Here's how the part is built. I have some questions about the finished solid (model axes, mm). Face numbers are marked on the shaded views. A direction names the side the tool comes from. Give positions to 0.01 mm unless a question says otherwise; leave off trailing zeros. Loops run counter-clockwise (first coordinate to the right, second up) from the corner with the lowest first, then second, coordinate; pieces in that order, holes last.
Q1. If we section it at B-B (z = 44.5): Please give me the cut outline in (x, y).
Q2. If we section it at C-C (x = 3): Please give me the cut outline in (y, z), plus the area to 3 significant figures.
Q3. I need wall thicknesses on line 1 (Z direction, x = 9.25, y = -12); line 2 (Y direction, x = 1.25, z = 5.5); line 3 (Y direction, x = 0.5, z = 43). Which ranges of each line are inside material? Lowest first, please.
Q4. Will these pins go through, and if not, where does the flat tip stop? P1, Ø3.5, axis at x = 7.5, z = -3, coming from the -Y side; P2, Ø5, axis at x = 8.5, z = 4.5, coming from the +Y side; P3, Ø3.5, axis at x = 0.5, z = -4, coming from the +Y side.
Q5. If we section it at A-A (y = -0.5): Please give me the cut outline in (x, z), plus the area to 3 significant figures.
Q6. For the marked faces 1, 2, 3 and 4, which set-ups out of +Z, -Z, +X, -X, +Y, -Y let a thin tool reach every point of the face, with its end or its side?
Q7. If we section it at D-D (z = 10): Please give me the cut outline in (x, y).
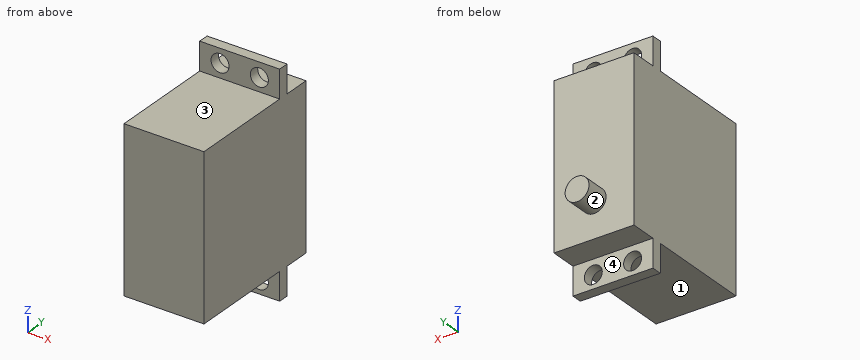
Autodesk Inventor part; units mm, degrees
ref_plane "YZ Plane" through (0, 0, 0) normal (1, 0, 0) x (0, 1, 0)
ref_plane "XZ Plane" through (0, 0, 0) normal (0, 1, 0) x (-1, 0, 0)
ref_plane "XY Plane" through (0, 0, 0) normal (0, 0, 1) x (1, 0, 0)
sketch "Sketch1" plane through (0, 0, 0) normal (0, 0, 1) x (1, 0, 0)
  line L0 (-7.4537, 7.1113) -> (12.5361, 7.1113)
  line L1 (12.5361, 7.1113) -> (12.5361, -28.8297)
  line L2 (12.5361, -28.8297) -> (-7.4537, -28.8297)
  line L3 (-7.4537, -28.8297) -> (-7.4537, 7.1113)
  point P0 (0, 0)
  dimension "d0" = 19.9898
  dimension "d1" = 35.941
extrude "Extrusion1" add sketch "Sketch1" along normal blind 40.386
sketch "Sketch2" plane through (0, 0, 0) normal (0, 0, -1) x (-1, 0, 0)
  line L0 (-12.5361, -28.8297) -> (-12.5361, 7.1113)
  line L1 (7.4537, -28.8297) -> (7.4537, 7.1113)
  line L2 (-12.5361, 0.4311) -> (7.4537, 0.4311)
  line L3 (7.4537, 0.4311) -> (7.4537, -2.1597)
  line L4 (7.4537, -2.1597) -> (-12.5361, -2.1597)
  line L5 (-12.5361, -2.1597) -> (-12.5361, 0.4311)
  line L6 (7.4537, 7.1113) -> (-12.5361, 7.1113)
  line L7 (-12.5361, -28.8297) -> (7.4537, -28.8297)
  line L8 (7.4537, 7.1113) -> (7.4537, -28.8297)
  line L9 (7.4537, 0.4311) -> (-12.5361, 0.4311)
  line L10 (-12.5361, 0.4311) -> (-12.5361, -2.1597)
  line L11 (-12.5361, -2.1597) -> (7.4537, -2.1597)
  line L12 (7.4537, -2.1597) -> (7.4537, 0.4311)
  point P0 (0, 0)
  dimension "d4" = 6.6802
  dimension "d5" = 2.5908
  dimension "d6" = 26.67
  dimension "d7" = 19.9898
  dimension "d8" = 2.5908
extrude "Extrusion2" add sketch "Sketch2" along normal blind 7.0104 contours L0 L2 L1 L4
sketch "Sketch3" plane through (0, 0, 40.386) normal (0, 0, 1) x (1, 0, 0)
  point P0 (0, 0)
sketch "Sketch4" plane through (0, 0, 40.386) normal (0, 0, 1) x (1, 0, 0)
  line L0 (-7.4537, -2.1597) -> (-7.4537, 0.4311)
  line L1 (12.5361, -2.1597) -> (-7.4537, -2.1597)
  line L2 (-7.4537, 0.4311) -> (12.5361, 0.4311)
  line L3 (12.5361, 0.4311) -> (12.5361, -2.1597)
  line L4 (12.5361, -2.1597) -> (-7.4537, -2.1597)
  line L5 (-7.4537, -2.1597) -> (-7.4537, 0.4311)
  point P0 (0, 0)
extrude "Extrusion3" add sketch "Sketch4" along normal blind 7.0104
sketch "Sketch5" plane through (-7.4537, 0.4311, 40.386) normal (0, 1, 0) x (1, 0, 0)
  circle A0 centre (14.9098, -3.3973) radius 2.2479
  line L0 (19.9898, 0) -> (19.9898, -7.0104)
  circle A1 centre (5.08, -3.5052) radius 2.2479
  line L1 (0, 0) -> (0, -7.0104)
  point P0 (7.4537, 40.386)
  dimension "d13" = 5.08
  dimension "d14" = 5.08
  dimension "d15" = 4.4958
  dimension "d16" = 4.4958
  dimension "d17" = 5.3346
sketch "Sketch6" plane through (-7.4537, 7.1113, 0) normal (0, 1, 0) x (1, 0, 0)
  point P0 (7.4537, 0)
sketch "Sketch7" plane through (-7.4537, 0.4311, 0) normal (0, 1, 0) x (1, 0, 0)
  circle A0 centre (14.9098, 3.6831) radius 2.2479
  circle A1 centre (5.08, 3.6831) radius 2.2479
  line L0 (19.9898, 0) -> (19.9898, 7.0104)
  line L1 (0, 0) -> (0, 7.0104)
  point P0 (7.4537, 0)
  dimension "d18" = 5.08
  dimension "d19" = 5.08
  dimension "d20" = 4.4958
  dimension "d21" = 4.4958
  dimension "d22" = 5.334
hole "Hole1" at (7.4561, 0.4311, 43.7833) at (-2.3737, 0.4311, 43.8912) direction (0, -1, 0) diameter 4.4958 end through all
hole "Hole2" at (7.4561, 0.4311, -3.6831) at (-2.3737, 0.4311, -3.6831) direction (0, -1, 0) diameter 4.4958 end through all
sketch "Sketch8" plane through (-7.4537, 7.1113, 0) normal (0, 1, 0) x (1, 0, 0)
  circle A0 centre (9.9711, -8.9281) radius 2.9845
  line L0 (0, 0) -> (19.9898, 0)
  point P0 (7.4537, 0)
  dimension "d37" = 5.9436
  dimension "d38" = 5.969
extrude "Extrusion4" add sketch "Sketch8" along normal blind 5.9944
sketch "Sketch9" plane through (0, 0, 0) normal (0, 0, -1) x (-1, 0, 0)
  point P0 (0, 0)
sketch "Sketch10" plane through (-7.4537, 7.1113, 0) normal (0, 1, 0) x (1, 0, 0)
  line L0 (0, 0) -> (19.9898, 0)
  line L1 (19.9898, 0) -> (19.9898, -40.386)
  line L2 (0, 0) -> (0, -40.386)
  line L3 (19.9898, -40.386) -> (0, -40.386)
  circle A0 centre (14.9098, -43.7833) radius 2.2479
  circle A1 centre (5.08, -43.8912) radius 2.2479
  circle A2 centre (14.9098, 3.6831) radius 2.2479
  circle A3 centre (5.08, 3.6831) radius 2.2479
  point P0 (7.4537, 0)
properties part number "RTS Motor"
Check sheet entries:
1. outline: (-7.45, -2.16) - (-4.54, -2.16) - (-4.54, 0.43) - (-7.45, 0.43) - close; (-0.21, -2.16) - (5.33, -2.16) - (5.33, 0.43) - (-0.21, 0.43) - close; (9.59, -2.16) - (12.54, -2.16) - (12.54, 0.43) - (9.59, 0.43) - close
2. outline: (-28.83, 0) - (-2.16, 0) - (-2.16, -7.01) - (0.43, -7.01) - (0.43, 0) - (7.11, 0) - (7.11, 5.98) - (13.11, 5.98) - (13.11, 11.87) - (7.11, 11.87) - (7.11, 40.39) - (0.43, 40.39) - (0.43, 47.4) - (-2.16, 47.4) - (-2.16, 40.39) - (-28.83, 40.39) - close
2. area: 1,520 mm2
3. line 1: z = 0 to 40.39
3. line 2: y = -28.83 to 7.11
3. line 3: y = -2.16 to 0.43
4. P1: stops at y = -2.16
4. P2: stops at y = 7.11
4. P3: stops at y = 0.43
5. outline: (-7.45, -7.01) - (12.54, -7.01) - (12.54, 47.4) - (-7.45, 47.4) - close; hole circle Ø4.5 at (-2.37, -3.68); hole circle Ø4.5 at (-2.37, 43.89); hole circle Ø4.5 at (7.46, -3.68); hole circle Ø4.5 at (7.46, 43.78)
5. area: 1,020 mm2
6. face 1: -Z, +X, -X, -Y
6. face 2: +Y
6. face 3: +Z, +X, -X, -Y
6. face 4: -Z, +X, -X, +Y
7. outline: (-7.45, -28.83) - (12.54, -28.83) - (12.54, 7.11) - (5.3, 7.11) - (5.3, 13.11) - (-0.27, 13.11) - (-0.27, 7.11) - (-7.45, 7.11) - close
